```python
from build123d import *

# Parameters (mm, degrees)
BOSS_EXTRUDE1_DEPTH = 15
SKETCH2_W           = 3
SKETCH2_H           = 0.5
BOSS_EXTRUDE2_DEPTH = 1
SKETCH3_W           = 3
SKETCH3_H           = 0.5
BOSS_EXTRUDE3_DEPTH = 1


with BuildPart() as part:
    # Sketch1 → Boss-Extrude1 (new body, symmetric)
    with BuildSketch(Plane.XY):
        Polygon((0, 0), (15, 0), (15, 32), (0, 32), (0, 31), (14, 31), (14, 1), (0, 1), align=None)
    extrude(amount=BOSS_EXTRUDE1_DEPTH, both=True)

    # Sketch2 → Boss-Extrude2 (add)
    with BuildSketch(Plane.ZY):
        with Locations((0, 31.5)):
            Rectangle(SKETCH2_W, SKETCH2_H)
    extrude(amount=BOSS_EXTRUDE2_DEPTH)

    # Sketch3 → Boss-Extrude3 (add)
    with BuildSketch(Plane.ZY):
        with Locations((0, 0.5)):
            Rectangle(SKETCH3_W, SKETCH3_H)
    extrude(amount=BOSS_EXTRUDE3_DEPTH)


solid = part.part
```
Geometry: final body of the model. Coordinates: model frame, mm. A direction names the side the tool comes from. Give positions to 0.01 mm unless a question says otherwise; leave off trailing zeros. Loops run counter-clockwise (first coordinate to the right, second up) from the corner with the lowest first, then second, coordinate; pieces in that order, holes last. Notation, with made-up numbers: (72, 49) - (113, 49) arc R28 cw to (113, 72) - close; hole circle Ø1 at (-12.75, 70). An arc over 180 degrees is marked (long way). Answer as CSV lines item,"result". Start each with the question number.
(1) Pin query (flat end, axial travel): P1, Ø0.8, axis at y = 0.5, z = -4, coming from the -X side; P2, Ø0.8, axis at x = -0.5, z = -0.5, coming from the +Y side; P3, Ø1.5, axis at y = 18, z = -12, coming from the -X side. Return the tip coordinate at first contact, or that it passes through.
(2) Reachability of faces 1 (the face through (-0.5, 31.75, 0)), 2 (the face through (-0.5, 0.25, 0)), 3 (the face through (14.7, 16.1, 15)), 4 (the face through (14, 16, 0)) from +Z, -Z, +X, -X, +Y, -Y: full face, straight path, thin tool, end or side. Return the list, or none.
(3) Section query D-D (z = 0.5). Output: boundary loops of the cut face in (x, y), and give its area (3 significant figures).
(4) Ray query, line 1 along Y through (x, z) = (7.75, -8.75); line 2 along X through (y, z) = (15.5, -9.5). Return the intervals inside material, ascending. Write a range as [from, to].
(5) Section query C-C (y = 2.5). Output: boundary loops of the cut face in (x, z), and give its area (3 significant figures).
(6) Section query B-B (z = -2.5). Output: boundary loops of the cut face in (x, y), and give its area (3 significant figures).
(7) Mould query, pull axis Y, two halves, no side actions, for faces 5 (the face through (8, 32, 0)), 6 (the face through (7, 31, 0)), 7 (the face through (15, 16, 0)). Classes: +Y half, -Y half, draft (parallel to the pull), parting line (faces both ways), or undercut.
(8) Section query A-A (x = 2). Output: boundary loops of the cut face in (y, z), and give its area (3 significant figures).
Worked answers:
1,P1,"stops at x = 0"
1,P2,"stops at y = 31.75"
1,P3,"stops at x = 14"
2,face 1,"+Z, -Z, -X, +Y"
2,face 2,"+Z, -Z, -X, -Y"
2,face 3,"+Z, +X, -X, +Y, -Y"
2,face 4,"+Z, -Z, -X"
3,outline,"(-1, 0.25) - (0, 0.25) - (0, 0) - (15, 0) - (15, 32) - (0, 32) - (0, 31.75) - (-1, 31.75) - (-1, 31.25) - (0, 31.25) - (0, 31) - (14, 31) - (14, 1) - (0, 1) - (0, 0.75) - (-1, 0.75) - close"
3,area,"61.0 mm^2"
4,line 1,"y = [0, 1], [31, 32]"
4,line 2,"x = [14, 15]"
5,outline,"(14, -15) - (15, -15) - (15, 15) - (14, 15) - close"
5,area,"30.0 mm^2"
6,outline,"(0, 0) - (15, 0) - (15, 32) - (0, 32) - (0, 31) - (14, 31) - (14, 1) - (0, 1) - close"
6,area,"60.0 mm^2"
7,face 5,"+Y half"
7,face 6,"undercut"
7,face 7,"draft"
8,outline,"(0, -15) - (1, -15) - (1, 15) - (0, 15) - close; (31, -15) - (32, -15) - (32, 15) - (31, 15) - close"
8,area,"60.0 mm^2"
